```python
from build123d import *

# Parameters (mm, degrees)
F1_DEPTH       = 6
F3_D           = 2.286
F3_DEPTH       = 3.302
F3_CSINK_D     = 4.191
F3_CSINK_ANGLE = 131
F3_TIP         = 0.6867836875
F4_D           = 2.286
F4_DEPTH       = 3.302
F4_CSINK_D     = 4.191
F4_CSINK_ANGLE = 131
F4_TIP         = 0.6867836875
F6_D           = 2.286
F6_DEPTH       = 31.75
F6_TIP         = 0.6867836875
F8_D           = 2.286
F8_DEPTH       = 31.75
F8_TIP         = 0.6867836875
F9_DEPTH       = 6


with BuildPart() as f1:
    # F0 (on Front) → F1 (new body)
    with BuildSketch(Plane.XZ):
        with BuildLine():
            Line((1, 16.5), (1, 6))
            Line((1, 6), (1, 0))
            Line((1, 0), (1, -6))
            Line((1, -6), (1, -16.5))
            Line((1, -16.5), (2, -16.5))
            ThreePointArc((2, -16.5), (2.7071067812, -16.2071067812), (3, -15.5))
            Line((3, -15.5), (3, -8.6602540378))
            ThreePointArc((3, -8.6602540378), (3.5001799931, -7.7941247399), (4.5003599214, -7.7944365345))
            Line((4.5003599214, -7.7944365345), (28.8345806574, -21.8572947335))
            Line((28.8345806574, -21.8572947335), (31.9750532508, -16.7448166758))
            Line((31.9750532508, -16.7448166758), (7.4946042855, -2.5974525099))
            ThreePointArc((7.4946042855, -2.5974525099), (5.9956840498, 0), (7.4946042855, 2.5974525099))
            Line((7.4946042855, 2.5974525099), (31.9750532508, 16.7448166758))
            Line((31.9750532508, 16.7448166758), (28.8345806574, 21.8572947335))
            Line((28.8345806574, 21.8572947335), (4.5003599214, 7.7944365345))
            ThreePointArc((4.5003599214, 7.7944365345), (3.5001799931, 7.7941247399), (3, 8.6602540378))
            Line((3, 8.6602540378), (3, 15.5))
            ThreePointArc((3, 15.5), (2.7071067812, 16.2071067812), (2, 16.5))
            Line((2, 16.5), (1, 16.5))
        make_face()
        with BuildLine():
            Line((-1, -6), (-1, 6))
            Line((-1, 6), (-1, 16.5))
            Line((-1, 16.5), (-3, 16.5))
            ThreePointArc((-3, 16.5), (-3.7071067812, 16.2071067812), (-4, 15.5))
            Line((-4, 15.5), (-4, -15.5))
            ThreePointArc((-4, -15.5), (-3.7071067812, -16.2071067812), (-3, -16.5))
            Line((-3, -16.5), (-1, -16.5))
            Line((-1, -16.5), (-1, -6))
        make_face()
        Polygon((1, 0), (1, 6), (-1, 6), (-1, -6), (1, -6), align=None)
    extrude(amount=F1_DEPTH)

    # F3
    with Locations(Plane(origin=(0, 0, 0), x_dir=(1, 0, 0), z_dir=(0, 1, 0))):
        with Locations((3, 3.4633801802)):
            CounterSinkHole(F3_D / 2, F3_CSINK_D / 2, depth=F3_DEPTH, counter_sink_angle=F3_CSINK_ANGLE)
            with Locations((0, 0, -(F3_DEPTH + F3_TIP / 2))):  # 118° drill point
                Cone(0, F3_D / 2, F3_TIP, mode=Mode.SUBTRACT)

    # F4
    with Locations(Plane(origin=(0, 0, 0), x_dir=(1, 0, 0), z_dir=(0, 1, 0))):
        with Locations((3, -3.4689440442)):
            CounterSinkHole(F4_D / 2, F4_CSINK_D / 2, depth=F4_DEPTH, counter_sink_angle=F4_CSINK_ANGLE)
            with Locations((0, 0, -(F4_DEPTH + F4_TIP / 2))):  # 118° drill point
                Cone(0, F4_D / 2, F4_TIP, mode=Mode.SUBTRACT)

    # F6
    with Locations(Plane(origin=(30.6831613521, 0, 18.8479297546), x_dir=(0, 1, 0), z_dir=(0.8520796763, 0, 0.5234120989))):
        with Locations((-3, 0.5317882384)):
            Hole(F6_D / 2, depth=F6_DEPTH)
            with Locations((0, 0, -(F6_DEPTH + F6_TIP / 2))):  # 118° drill point
                Cone(0, F6_D / 2, F6_TIP, mode=Mode.SUBTRACT)

    # F8
    with Locations(Plane(origin=(30.6831613521, 0, -18.8479297546), x_dir=(0, 1, 0), z_dir=(0.8520796763, 0, -0.5234120989))):
        with Locations((-3, -0.5317882384)):
            Hole(F8_D / 2, depth=F8_DEPTH)
            with Locations((0, 0, -(F8_DEPTH + F8_TIP / 2))):  # 118° drill point
                Cone(0, F8_D / 2, F8_TIP, mode=Mode.SUBTRACT)

    # F0 (on Front) → F9 (join)
    with BuildSketch(Plane.XZ):
        with BuildLine():
            ThreePointArc((31.9750532508, 16.7448166758), (33.0305925786, 20.9140066634), (28.8345806574, 21.8572947335))
            Line((28.8345806574, 21.8572947335), (31.9750532508, 16.7448166758))
        make_face()
        with BuildLine():
            Line((31.9750532508, -16.7448166758), (28.8345806574, -21.8572947335))
            ThreePointArc((28.8345806574, -21.8572947335), (32.8933608768, -20.829708522), (31.9750532508, -16.7448166758))
        make_face()
    extrude(amount=F9_DEPTH)


solid = f1.part
```
Geometry: final body of the model. Coordinates: model frame, mm. A direction names the side the tool comes from. Round coordinates to 2 decimals unless told otherwise and drop trailing zeros. Loops run counter-clockwise (first coordinate to the right, second up) from the corner with the lowest first, then second, coordinate; pieces in that order, holes last.
Item 1: Line query: L1, parallel to Z at x = 29, y = -2.5; L2, parallel to Y at x = 18, z = -11.5; L3, parallel to X at y = -3.8, z = 15.5. Output: solid intervals per line, ascending.
Checked values:
L1: z = -21.95 to -19.64, -17.23 to -15.03, 15.03 to 17.23, 19.64 to 21.96
L2: y = -6 to -4.13, -1.87 to 0
L3: x = -4 to -1, 1 to 3, 17.83 to 22.66, 25.78 to 29.82
Item 2: Section B-B, the plane x = 17. State how many separate pieces and enclosed holes the cut face has, plus the area to 3 significant figures.
Checked values:
separate pieces: 2
enclosed holes: 2
area: 73.5 mm2
Item 3: Contact query for flat-ended pins moving along their axis: P1, Ø1.8, axis at x = 3, z = -3.46, coming from the +Y side; P2, Ø2, axis at x = -2, y = -1.5, coming from the -Z side; P3, Ø3, axis at y = -4, z = 11, coming from the +X side. Output: stop coordinate, or through.
Checked values:
P1: stops at y = -3.45
P2: stops at z = -16.5
P3: stops at x = 24.63
Item 4: Mould query, pull axis Z, two halves, no side actions, for faces 5 (the cylindrical face through (-3.715, -2.958, -16.199)), 6 (the cylindrical face through (5.996, -2.958, -0.044)), 7 (the flat face through (-1, -3, 11)). Classes: released by +Z, released by -Z, zero draft, split by the parting line, or undercut.
Checked values:
face 5: released by -Z
face 6: undercut
face 7: zero draft
Item 5: Reachability of faces 1 (the flat face through (-1, -3, -11)), 2 (the cylindrical face through (2.715, -2.958, 16.199)), 3 (the flat face through (1.5, -3, 16.5)), 4 (the flat face through (30.4, -2.98, 19.31)) from +Z, -Z, +X, -X, +Y, -Y: full face, straight path, thin tool, end or side. Return the list, or none.
Checked values:
face 1: -Z, +Y, -Y
face 2: +Z, +Y, -Y
face 3: +Z, -X, +Y, -Y
face 4: none
Item 6: Section A-A, the plane y = -1.1. Output: boundary loops of the cut face in (x, z), plus the area to 3 significant figures.
Checked values:
outline: (-4, -15.5) arc R1 ccw to (-3, -16.5) - (-1, -16.5) - (-1, -6) - (1, -6) - (1, -16.5) - (2, -16.5) arc R1 ccw to (3, -15.5) - (3, -8.66) arc R1 cw to (4.5, -7.79) - (28.83, -21.86) arc R3 ccw to (31.98, -16.74) - (7.49, -2.6) arc R3 cw to (7.49, 2.6) - (31.98, 16.74) arc R3 ccw (long way) to (28.83, 21.86) - (4.5, 7.79) arc R1 cw to (3, 8.66) - (3, 15.5) arc R1 ccw to (2, 16.5) - (1, 16.5) - (1, 6) - (-1, 6) - (-1, 16.5) - (-3, 16.5) arc R1 ccw to (-4, 15.5) - close; hole circle Ø2.29 at (3, -3.46); hole circle Ø2.29 at (3, 3.47)
area: 595 mm2
